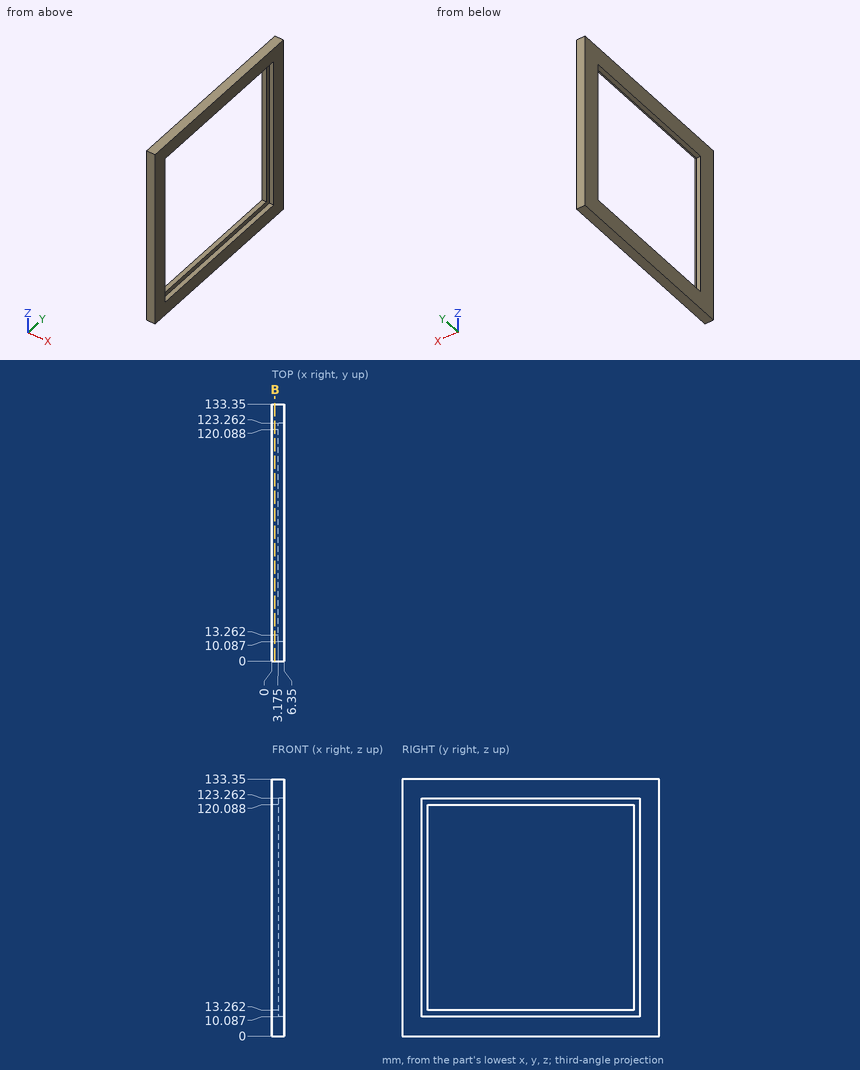
Design review of the part shown in the three views and the two pictorial views. Dimensions are in mm from the part's minimum x, y and z. Give positions to 0.01 mm unless a question says otherwise; leave off trailing zeros. Write each loop counter-clockwise with the first axis right and the second up, starting at its lowest first coordinate (ties: lowest second). Pieces come first, ordered by that corner, then holes.
Item 1: Wall thickness on probe 1 along Z at (x, y) = (4.5, 13.5); probe 2 along Y at (x, z) = (1.75, 118): over which ranges is each line inside the solid? List them lowest first.
Item 2: Take a section at B-B (x = 1.5). Give the boundary of the cut face in (y, z), and give its area (3 significant figures).
Item 3: Insertion check: P1, Ø3.5, axis at x = 4.5, y = 90, coming from the -Z side. The pin has a flat end and moves straight along its axis. Give the tip position at first contact, or say it passes through.
Established:
1. probe 1: z = 0 to 10.09, 123.26 to 133.35
1. probe 2: y = 0 to 13.26, 120.09 to 133.35
2. outline: (0, 0) - (133.35, 0) - (133.35, 133.35) - (0, 133.35) - close; hole (13.26, 13.26) - (120.09, 13.26) - (120.09, 120.09) - (13.26, 120.09) - close
2. area: 6,370 mm2
3. P1: stops at z = 0
